```python
from build123d import *

# Parameters (mm, degrees)
SKETCH1_W           = 60
SKETCH1_H           = 20
BOSS_EXTRUDE1_DEPTH = 5
SKETCH2_W           = 15
SKETCH2_H           = 5
CUT_EXTRUDE1_DEPTH  = 5
SKETCH3_W           = 60
SKETCH3_H           = 50
BOSS_EXTRUDE2_DEPTH = 5
SKETCH4_W           = 25
SKETCH4_H           = 50
BOSS_EXTRUDE3_DEPTH = 5
SKETCH5_W           = 25
SKETCH5_H           = 50
BOSS_EXTRUDE4_DEPTH = 5
SKETCH7_W           = 10
SKETCH7_H           = 50
BOSS_EXTRUDE5_DEPTH = 5
SKETCH8_W           = 10
SKETCH8_H           = 50
BOSS_EXTRUDE6_DEPTH = 5
SKETCH9_W           = 70
SKETCH9_H           = 5.5
BOSS_EXTRUDE8_DEPTH = 5
SKETCH11_W          = 70
SKETCH11_H          = 20
BOSS_EXTRUDE9_DEPTH = 5


with BuildPart() as part:
    # Sketch1 → Boss-Extrude1 (new body)
    with BuildSketch(Plane(origin=(0, 0, 0), x_dir=(1, 0, 0), z_dir=(0, 1, 0))):
        Rectangle(SKETCH1_W, SKETCH1_H)
    extrude(amount=BOSS_EXTRUDE1_DEPTH)

    # Sketch2 → Cut-Extrude1 (cut)
    with BuildSketch(Plane(origin=(0, 5, 0), x_dir=(1, 0, 0), z_dir=(0, 1, 0))):
        with Locations((-16.5, 3.5)):
            Rectangle(SKETCH2_W, SKETCH2_H)
    extrude(amount=-CUT_EXTRUDE1_DEPTH, mode=Mode.SUBTRACT)

    # Sketch3 → Boss-Extrude2 (add)
    with BuildSketch(Plane(origin=(0, 0, -10), x_dir=(-1, 0, 0), z_dir=(0, 0, -1))):
        with Locations((0, 25)):
            Rectangle(SKETCH3_W, SKETCH3_H)
    extrude(amount=BOSS_EXTRUDE2_DEPTH)

    # Sketch4 → Boss-Extrude3 (add)
    with BuildSketch(Plane(origin=(30, 0, 0), x_dir=(0, 0, -1), z_dir=(1, 0, 0))):
        with Locations((2.5, 25)):
            Rectangle(SKETCH4_W, SKETCH4_H)
    extrude(amount=BOSS_EXTRUDE3_DEPTH)

    # Sketch5 → Boss-Extrude4 (add)
    with BuildSketch(Plane.ZY.offset(30)):
        with Locations((-2.5, 25)):
            Rectangle(SKETCH5_W, SKETCH5_H)
    extrude(amount=BOSS_EXTRUDE4_DEPTH)

    # Sketch7 → Boss-Extrude5 (add)
    with BuildSketch(Plane.XY.offset(10)):
        with Locations((30, 25)):
            Rectangle(SKETCH7_W, SKETCH7_H)
    extrude(amount=BOSS_EXTRUDE5_DEPTH)

    # Sketch8 → Boss-Extrude6 (add)
    with BuildSketch(Plane.XY.offset(10)):
        with Locations((-30, 25)):
            Rectangle(SKETCH8_W, SKETCH8_H)
    extrude(amount=BOSS_EXTRUDE6_DEPTH)

    # Sketch9 → Boss-Extrude8 (add)
    with BuildSketch(Plane(origin=(0, 50, 0), x_dir=(1, 0, 0), z_dir=(0, 1, 0))):
        with Locations((0, 17.75)):
            Rectangle(SKETCH9_W, SKETCH9_H)
    extrude(amount=-BOSS_EXTRUDE8_DEPTH)

    # Sketch11 → Boss-Extrude9 (add)
    with BuildSketch(Plane(origin=(0, 0, -20.5), x_dir=(-1, 0, 0), z_dir=(0, 0, -1))):
        with Locations((0, 40)):
            Rectangle(SKETCH11_W, SKETCH11_H)
    extrude(amount=BOSS_EXTRUDE9_DEPTH)


solid = part.part
```
Model file for the job. Use its own axes, mm. A direction names the side the tool comes from. Give positions to 0.01 mm unless a question says otherwise; leave off trailing zeros. Write each loop counter-clockwise with the first axis right and the second up, starting at its lowest first coordinate (ties: lowest second). Pieces come first, ordered by that corner, then holes. Notation, with made-up numbers: M 29,-8 L 68,-8 A25 cw 68,19 Z; hole C 44.5,-38 d11. An arc over 180 degrees is marked long. Use a Markdown table: item, result.
1) Drill centre lines: line 1 (Z direction, x = 26, y = 43.5); line 2 (Z direction, x = 29, y = 18); line 3 (X direction, y = 16, z = 6). Where is each one in solid material? Low to high. Write a range as from..to.
Responses:
| item | result |
|---|---|
| line 1 | z = -25.5..-20.5, -15..-10, 10..15 |
| line 2 | z = -15..-10, 10..15 |
| line 3 | x = -35..-30, 30..35 |
2) Cut at C-C (y = 37). List the corners of the cut face in (x, z), and give its area (3 significant figures).
Responses:
| item | result |
|---|---|
| outline | M -35,-25.5 L 35,-25.5 L 35,-20.5 L -35,-20.5 Z; M -35,-15 L 35,-15 L 35,15 L 25,15 L 25,10 L 30,10 L 30,-10 L -30,-10 L -30,10 L -25,10 L -25,15 L -35,15 Z |
| area | 1,000 mm2 |
3) Cut at D-D (z = 4.5). List the corners of the cut face in (x, y), and give its area (3 significant figures).
Responses:
| item | result |
|---|---|
| outline | M -35,0 L 35,0 L 35,50 L 30,50 L 30,5 L -30,5 L -30,50 L -35,50 Z |
| area | 800 mm2 |
4) Tool access for faces 1 (the flat face through (0, 28, -10)), 2 (the flat face through (-24, 3, -3)), 3 (the flat face through (25, 25, 12)), 4 (the flat face through (0, 22, -15)), 5 (the flat face through (0, 30, -23)): list every direction of +Z, -Z, +X, -X, +Y, -Y with a clear straight run to the whole face (end or side of a thin tool).
Responses:
| item | result |
|---|---|
| face 1 | +Y |
| face 2 | +Y, -Y |
| face 3 | +Z, +Y, -Y |
| face 4 | +X, -X, -Y |
| face 5 | -Z, +X, -X, -Y |
5) Cut at B-B (z = -4.5). List the corners of the cut face in (x, y).
Responses:
| item | result |
|---|---|
| outline | M -35,0 L -24,0 L -24,5 L -30,5 L -30,50 L -35,50 Z; M -9,0 L 35,0 L 35,50 L 30,50 L 30,5 L -9,5 Z |
6) Cut at A-A (x = -11). List the corners of the cut face in (y, z).
Responses:
| item | result |
|---|---|
| outline | M 0,-15 L 45,-15 L 45,-20.5 L 30,-20.5 L 30,-25.5 L 50,-25.5 L 50,-10 L 5,-10 L 5,-6 L 0,-6 Z; M 0,-1 L 5,-1 L 5,10 L 0,10 Z |
7) Pin check, flat tips, straight feed: pin 1 (22 mm diameter, centred on x = 9.5, z = 2, fed in from +Y); pin 2 (5.5 mm diameter, centred on x = -17.5, y = 1.5, fed in from -Z); pin 3 (7.5 mm diameter, centred on x = 8.5, y = 37, fed in from +Z). Stop position of each tip, or through.
Responses:
| item | result |
|---|---|
| pin 1 | stops at y = 5 |
| pin 2 | stops at z = -15 |
| pin 3 | stops at z = -10 |
8) Pull direction Z, two halves, no side cores. Call faces 6 (the flat face through (-30, 25, 15)), 7 (the flat face through (0, 0, 0)), 8 (the flat face through (-17, 3, -6)): +Z half, -Z half, draft (parallel to the pull), parting line (faces both ways), or undercut.
Responses:
| item | result |
|---|---|
| face 6 | +Z half |
| face 7 | draft |
| face 8 | undercut |
